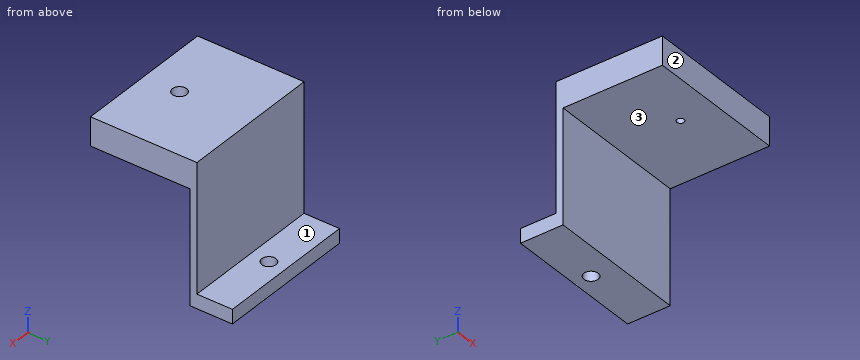
from build123d import *

# Parameters (mm, degrees)
F1_DEPTH       = 1000
F3_D           = 100
F5_D           = 50
F5_CBORE_D     = 100
F5_CBORE_DEPTH = 100


with BuildPart() as f1:
    # F0 (on Right) → F1 (new body)
    with BuildSketch(Plane.YZ):
        Polygon((-300, 0), (0, 0), (0, 100), (-250, 100), (-250, 1000), (-1000, 1000), (-1000, 800), (-300, 800), align=None)
    extrude(amount=F1_DEPTH)

    # F3 (through all)
    with Locations(Plane.XY.offset(100)):
        with Locations((500, -120)):
            Hole(F3_D / 2)

    # F5 (through all)
    with Locations(Plane.XY.offset(1000)):
        with Locations((500, -750)):
            CounterBoreHole(F5_D / 2, F5_CBORE_D / 2, F5_CBORE_DEPTH)


solid = f1.part
Work out the finished part from the listing and answer in its coordinate system (mm). Face numbers are marked on the shaded views. A direction names the side the tool comes from. Round coordinates to 2 decimals unless told otherwise and drop trailing zeros. Write each loop counter-clockwise with the first axis right and the second up, starting at its lowest first coordinate (ties: lowest second). Pieces come first, ordered by that corner, then holes.
1) A cutting plane is placed at B-B (z = 938). Give the vertices of the cut face in (x, y).
2) A cutting plane is placed at A-A (y = -750). Give the vertices of the cut face in (x, z), plus the area to 3 significant figures.
3) Straight lines are drawn through the part: line 1 (Y direction, x = 500, z = 879.5); line 2 (Y direction, x = 500, z = 55.5); line 3 (Z direction, x = 669, y = -209.5). For each, find the intervals that lie inside material, in ascending order.
4) A cutting plane is placed at D-D (x = 88). Give the vertices of the cut face in (y, z).
5) A cutting plane is placed at C-C (x = 500). Give the vertices of the cut face in (y, z), plus the area to 3 significant figures.
6) Given pin 1 Ø8 at (x, y) = (301.5, -124) entering from -Z; pin 2 Ø12 at (x, z) = (385, 454) entering from -Y; pin 3 Ø5 at (x, z) = (469.5, 669.5) entering from +Y, each flat-ended and moving along its own axis, determine where each tip first touches the part or whether it passes through.
7) A tool of negligible diameter and unlimited length cuts with its end or side. For the marked faces 1, 2 and 3, from which of +Z, -Z, +X, -X, +Y, -Y can it reach the whole face along a straight path? Write none if from no direction.
Completed:
1. outline: (0, -1000) - (1000, -1000) - (1000, -250) - (0, -250) - close; hole circle Ø100 at (500, -750)
2. outline: (0, 800) - (475, 800) - (475, 900) - (450, 900) - (450, 1000) - (0, 1000) - close; (525, 800) - (1000, 800) - (1000, 1000) - (550, 1000) - (550, 900) - (525, 900) - close
2. area: 185,000 mm2
3. line 1: y = -1000 to -775, -725 to -250
3. line 2: y = -300 to -170, -70 to 0
3. line 3: z = 0 to 100
4. outline: (-1000, 800) - (-300, 800) - (-300, 0) - (0, 0) - (0, 100) - (-250, 100) - (-250, 1000) - (-1000, 1000) - close
5. outline: (-1000, 800) - (-775, 800) - (-775, 900) - (-800, 900) - (-800, 1000) - (-1000, 1000) - close; (-725, 800) - (-300, 800) - (-300, 0) - (-170, 0) - (-170, 100) - (-250, 100) - (-250, 1000) - (-700, 1000) - (-700, 900) - (-725, 900) - close; (-70, 0) - (0, 0) - (0, 100) - (-70, 100) - close
5. area: 190,000 mm2
6. pin 1: stops at z = 0
6. pin 2: stops at y = -300
6. pin 3: stops at y = -250
7. face 1: +Z, +X, -X, +Y
7. face 2: +Z, -Z, +X, -X, -Y
7. face 3: -Z, +X, -X, -Y
